```python
from build123d import *

# Parameters (mm, degrees)
AUFSATZ_LINEAR_AUSTRAGEN1_DEPTH      = 9.8
AUFSATZ_LINEAR_AUSTRAGEN1_DEPTH_BACK = 9.8
SKIZZE1_R                            = 9.6
SKIZZE2_R                            = 11.1
AUFSATZ_LINEAR_AUSTRAGEN2_DEPTH      = 1.4
AUFSATZ_LINEAR_START                 = -1.4
SKIZZE3_R                            = 11.1
AUFSATZ_LINEAR_AUSTRAGEN3_DEPTH      = 1.4
FASE1_SIZE                           = 0.5


with BuildPart() as part:
    # Skizze1 → Aufsatz-Linear austragen1 (new, two sides: drawn at the far end of the back side and taken through both)
    with BuildSketch(Plane.XY.offset(-AUFSATZ_LINEAR_AUSTRAGEN1_DEPTH_BACK)):
        Circle(SKIZZE1_R)
    extrude(amount=AUFSATZ_LINEAR_AUSTRAGEN1_DEPTH + AUFSATZ_LINEAR_AUSTRAGEN1_DEPTH_BACK)

    # Skizze2 → Aufsatz-Linear austragen2 (add)
    with BuildSketch(Plane.XY.offset(9.8)):
        Circle(SKIZZE2_R)
    extrude(amount=-AUFSATZ_LINEAR_AUSTRAGEN2_DEPTH)

    # Skizze3 → Aufsatz-Linear austragen3 (add)
    with BuildSketch(Plane(origin=(0, 0, -9.8), x_dir=(-1, 0, 0), z_dir=(0, 0, -1)).offset(AUFSATZ_LINEAR_START)):
        with Locations(Location((0, 0, 0), (0, 0, 180))):
            Circle(SKIZZE3_R)
    extrude(amount=AUFSATZ_LINEAR_AUSTRAGEN3_DEPTH)

    # Skizze8 → Schnitt-Rotation1 (revolve, cut)
    with BuildSketch(Plane(origin=(0, 0, 0), x_dir=(0, 0, -1), z_dir=(1, 0, 0)), mode=Mode.PRIVATE) as schnitt_rotation1_sk:
        Polygon((9.8, 0), (9.8, 8), (8.4, 8), (-2.2, 4), (-2.2, 2.691026714), (-5.8, 2.691026714), (-5.8, 4.1), (-9.8, 4.1), (-9.8, 0), align=None)
    revolve(schnitt_rotation1_sk.sketch.rotate(Axis((0, 0, -9.8), (0, 0, 1)), 90), axis=Axis((0, 0, -9.8), (0, 0, 1)), mode=Mode.SUBTRACT)

    # Fase1
    fase1_edges = [part.edges().sort_by_distance(p)[0] for p in [
        (2.691026714, 0, 2.2),
        (2.691026714, 0, 5.8),
        (4.1, 0, 9.8),
    ]]
    chamfer(fase1_edges, length=FASE1_SIZE)


solid = part.part
```
Could you check a few things on this model? Use its own coordinates, in mm. A direction names the side the tool comes from. Round coordinates to 2 decimals unless told otherwise and drop trailing zeros. Loops run counter-clockwise (first coordinate to the right, second up) from the corner with the lowest first, then second, coordinate; pieces in that order, holes last. Notation, with made-up numbers: (2, 49.25) -> (17, 49.25) arc R26 ccw to (17, 88.25) -> close; hole circle Ø4 at (12, 11). An arc over 180 degrees is marked (long way). Put each result on its own line as item: value.
Q1. I want a section at D-D on x = 9.25. Write out the boundary of the cut face in (y, z).
Checks:
outline: (-6.14, -9.8) -> (6.14, -9.8) -> (6.14, -8.4) -> (2.57, -8.4) -> (2.57, 8.4) -> (6.14, 8.4) -> (6.14, 9.8) -> (-6.14, 9.8) -> (-6.14, 8.4) -> (-2.57, 8.4) -> (-2.57, -8.4) -> (-6.14, -8.4) -> close
Q2. Please list where these lines run through material, in increasing order: line 1 (Y direction, x = 0, z = 3.45); line 2 (Z direction, x = 6.25, y = 8.5); line 3 (Y direction, x = 0, z = -9.3). Write a range as from..to.
Checks:
line 1: -9.6..-2.69, 2.69..9.6
line 2: -9.8..-8.4, 8.4..9.8
line 3: -11.1..-8, 8..11.1
Q3. Which directions (+Z, -Z, +X, -X, +Y, -Y) give clear straight access to the entire face, cutting with the end or side of a thin tool? Please do faces 4 (the flat face through (-7, 7, 8.4)), 5 (the flat face through (3, 2, 2.2)), 6 (the cylindrical face through (0.534, -4.065, 7.574)).
Checks:
face 4: none
face 5: -Z
face 6: +Z
Q4. For pin 1 Ø4 at (x, y) = (-2, 1) entering from +Z; pin 2 Ø10 at (x, z) = (5, -1.5) entering from +Y; pin 3 Ø1.5 at (y, z) = (3.5, 2) entering from -X, each with a flat end and sliding along its axis, tell me the tip position at first contact or that it passes through.
Checks:
pin 1: z = 9.44
pin 2: y = 9.6
pin 3: x = -9.2
Q5. Thinking about a two-plate mould opening in X: for faces 1 (the flat face through (6, -6, -9.8)), 2 (the cylindrical face through (1.73, 7.81, -9.09)), 3 (the cylindrical face through (-1.445, -11.006, -9.09)), which applies, pulls with the +X half, pulls with the -X half, needs draft (parallel to the pull), parting line crosses it, or undercut?
Checks:
face 1: needs draft
face 2: undercut
face 3: parting line crosses it
Q6. I want a section at C-C on z = 8.75. Write out the boundary of the cut face in (x, y).
Checks:
outline: circle Ø22.2 at (0, 0); hole circle Ø8.2 at (0, 0)
